Autodesk Inventor part; units mm, degrees
sketch "Skizze1" plane through (0, 0, 0) normal (0, 0, 1) x (1, 0, 0)
  line L0 (4, 3.3) -> (0, 2.5)
  line L1 (4.5, 4.9297) -> (0, 4.0297)
  line L2 (0, 2.5) -> (0, 4.0297)
  line L3 (4.5, 4.9297) -> (4.5, 3.4)
  line L4 (-0.9, 0) -> (5.4, 0)
  line L5 (4.5, 3.4) -> (4.5, 0)
  line L6 (4, 3.3) -> (4, 0)
  line L7 (4, 0) -> (4.5, 0)
  point P0 (0, 0)
  dimension "d53" = 2.5
  dimension "d55" = 1.5
  dimension "d61" = 4.5
  dimension "d62" = 0.5
revolve "Umdrehung1" add sketch "Skizze1" angle 360 about axis through (-10, 0, 0) along (1, 0, 0)
fillet "Rundung8" radius 1.5 1 edges at (0, -2.5, 0)
fillet "Rundung9" radius 0.25 1 edges at (4.5, -4.9297, 0)
properties part number "ScheinwerferFront"
Can you work these out from the model? Positions are in its coordinate system, mm. Give positions to 0.01 mm unless a question says otherwise; leave off trailing zeros. Loops run counter-clockwise (first coordinate to the right, second up) from the corner with the lowest first, then second, coordinate; pieces in that order, holes last. Notation, with made-up numbers: (-21, 11.5) -> (13, 11.5) arc R20 ccw to (13, 40.5) -> close; hole circle Ø10 at (-2, -3.75). An arc over 180 degrees is marked (long way). Write item = value, one per line.
1) I need wall thicknesses on L1, parallel to Y at x = 1.55, z = 0.75; L2, parallel to Z at x = 2.4, y = 0; L3, parallel to Z at x = 1.2, y = 1.5. Which ranges of each line are inside material? Lowest first, please. Write a range as from..to.
Check result:
L1 = -4.27..-2.72, 2.72..4.27
L2 = -4.51..-2.98, 2.98..4.51
L3 = -4..-2.42, 2.42..4
2) Suppose I cut it at A-A on y = 0. Write out the boundary of the cut face in (x, z), then the cut area to 3 significant figures.
Check result:
outline = (0, -4.03) -> (4.2, -4.87) arc R0.25 ccw to (4.5, -4.62) -> (4.5, 4.62) arc R0.25 ccw to (4.2, 4.87) -> (0, 4.03) arc R1.5 ccw to (1.77, 2.85) -> (4, 3.3) -> (4, -3.3) -> (1.77, -2.85) arc R1.5 ccw to start
area = 15.7 mm2
3) Suppose I cut it at D-D on x = 2.9. Write out the boundary of the cut face in (y, z), then the cut area to 3 significant figures.
Check result:
outline = circle Ø9.22 at (0, 0); hole circle Ø6.16 at (0, 0)
area = 37.0 mm2
4) Suppose I cut it at B-B on x = 3.5. Write out the boundary of the cut face in (y, z).
Check result:
outline = circle Ø9.46 at (0, 0); hole circle Ø6.4 at (0, 0)
5) Thinking about a two-plate mould opening in Y: for faces 1 (the conical face through (2.402, -2.977, 0.131)), 2 (the flat face through (4.5, 0, 0)), 3 (the flat face through (4, 0, 0)), 4 (the conical face through (1.196, 4.072, 1.282)), which applies, released by +Y, released by -Y, zero draft, split by the parting line, or undercut?
Check result:
face_1 = undercut
face_2 = zero draft
face_3 = undercut
face_4 = split by the parting line
6) Will these pins go through, and if not, where does the flat tip stop? pin 1 (2 mm diameter, centred on y = 3, z = 0.5, fed in from -X); pin 2 (3.5 mm diameter, centred on y = -0.5, z = -0.5, fed in from -X); pin 3 (1.5 mm diameter, centred on x = 1.5, z = 2.5, fed in from +Y).
Check result:
pin_1 = 0
pin_2 = 4
pin_3 = 4
